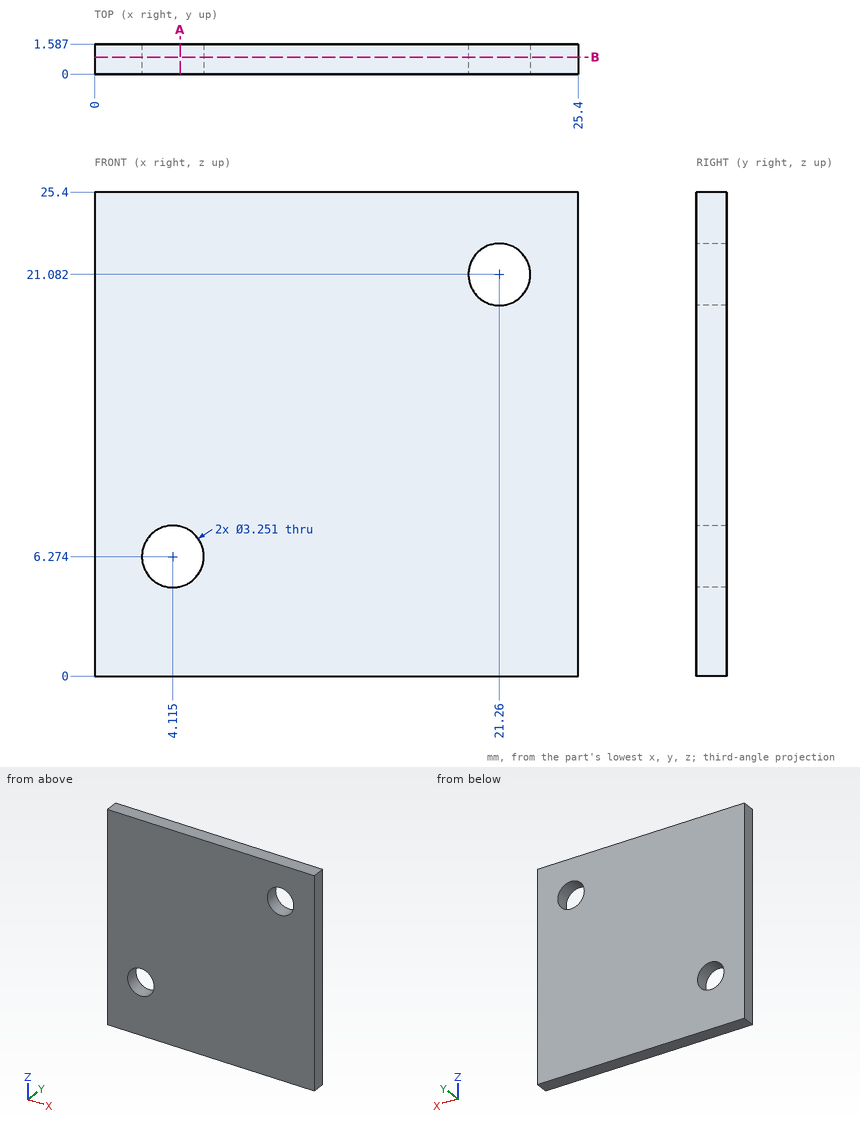
Answer from the drawing. Dimensions are ordinates in mm from the lowest x, y and z of the part. Coordinates: 2 decimals unless noted, no trailing zeros. Write each loop counter-clockwise with the first axis right and the second up, starting at its lowest first coordinate (ties: lowest second). Pieces come first, ordered by that corner, then holes. Notation, with made-up numbers: M 69,69 L 85,69 A12 cw 85,91 Z; hole C 1.5,43 d7. An arc over 180 degrees is marked long. Put each result on its own line as item: value. Start each with the question number.
1. A cutting plane is placed at B-B on y = 0.9. Write down the section's boundary in (x, z) (1 decimal).
2. Consider line 1 (Z direction, x = 21.25, y = 1.35); line 2 (X direction, y = 0.35, z = 20.75); line 3 (Z direction, x = 20, y = 0.4) (1 decimal). Determine where each line is inside the solid, lowest interval first. Write a range as from..to.
3. A flat-ended cylindrical pin translates along its axis: P1, Ø4, axis at x = 21.26, z = 21.08, coming from the +Y side. Find the tip coordinate at first contact, or state that the pin passes through.
4. A cutting plane is placed at A-A on x = 4.5. Write down the section's boundary in (y, z) (1 decimal).
Resolved:
1. outline: M 0,0 L 25.4,0 L 25.4,25.4 L 0,25.4 Z; hole C 4.1,6.3 d3.3; hole C 21.3,21.1 d3.3
2. line 1: z = 0..19.46, 22.71..25.4
2. line 2: x = 0..19.67, 22.85..25.4
2. line 3: z = 0..20.1, 22.1..25.4
3. P1: stops at y = 1.59
4. outline: M 0,0 L 1.6,0 L 1.6,4.7 L 0,4.7 Z; M 0,7.9 L 1.6,7.9 L 1.6,25.4 L 0,25.4 Z
